Design review of the part built by this model. Coordinates are the model's own, in mm. A direction names the side the tool comes from. Coordinates: 2 decimals unless noted, no trailing zeros. Loops run counter-clockwise (first coordinate to the right, second up) from the corner with the lowest first, then second, coordinate; pieces in that order, holes last. Notation, with made-up numbers: (45, -33.5) -> (93, -33.5) arc R21 cw to (93, -4.5) -> close; hole circle Ø5 at (5, 40.5). An arc over 180 degrees is marked (long way). Use a Markdown table: item, result. Add a question column.
Q1. Take a section at B-B on y = -89.5. Write out the cut boundary in (x, z), plus the area to 3 significant figures.
Q2. Take a section at A-A on x = -114.5. Write out the cut boundary in (y, z), plus the area to 3 significant figures.
Q3. Clearance check with flat-ended pins moving along their axes: pin 1 Ø7 at (x, y) = (-122.68, -90.83) entering from -Z; pin 2 Ø7.5 at (y, z) = (-76.5, 57) entering from +X; pin 3 Ø1.5 at (x, z) = (-116.5, 21) entering from -Y; pin 4 Ø1.5 at (y, z) = (-89.5, 55.5) entering from +X. State where each tip first meets the part, or that it passes through.
Q4. For faces 4 (the face through (-111, -96.022, 39)), 5 (the face through (-127.874, -79, 39)), 6 (the face through (-123.036, -88.155, 39.44)), list the 3-axis set-ups (+Z, -Z, +X, -X, +Y, -Y) from which the entire face can be reached by the end or side of a thin tool; tool diameter is ignored.
Q5. For probe 1 along Y at (x, z) = (-122.75, 10.5); probe 2 along Y at (x, z) = (-111.75, 23); probe 3 along X at (y, z) = (-90, 36), list the stretches that pass through material, from the lowest coordinate up.
Q6. Take a section at D-D on x = -132.75. Write out the cut boundary in (y, z), plus the area to 3 significant figures.
Q7. Take a section at C-C on z = 11.5. Write out the cut boundary in (x, y), plus the area to 3 significant figures.
Q8. Draft analysis for pull direction Y (two halves, no side actions). For faces 1 (the face through (-132, -74.122, 39)), 2 (the face through (-115.974, -98, 39)), 3 (the face through (-121, -86, 0)), state which applies: pulls with the +Y half, pulls with the -Y half, needs draft (parallel to the pull), parting line crosses it, or undercut.
from build123d import *

# Parameters (mm, degrees)
F0_R        = 2.7
F1_DEPTH    = 80
F2_T1_DEPTH = 91.0076112648


# Not quite as in the source:
# - a fillet or chamfer that OpenCascade refuses, or shapes differently, is made with other operations: its cross-section is extruded or revolved along the edge and cut away or added


with BuildPart() as f1:
    # F0 (on Top) → F1 (new body)
    with BuildSketch(Plane.XY):
        with BuildLine():
            Line((-130.9739977717, -74.1217002273), (-135.9739977717, -74.1217002273))
            ThreePointArc((-135.9739977717, -74.1217002273), (-127.1872012073, -95.3349036629), (-105.9739977717, -104.1217002273))
            Line((-105.9739977717, -104.1217002273), (-105.9739977717, -99.1217002273))
            Line((-105.9739977717, -99.1217002273), (-115.4739977717, -99.1217002273))
            ThreePointArc((-115.4739977717, -99.1217002273), (-116.3275511623, -99.4752536179), (-115.9739977717, -98.6217002273))
            Line((-115.9739977717, -98.6217002273), (-115.9739977717, -96.5217002273))
            ThreePointArc((-115.9739977717, -96.5217002273), (-116.3275511623, -95.6681468367), (-115.4739977717, -96.0217002273))
            Line((-115.4739977717, -96.0217002273), (-105.9739977717, -96.0217002273))
            Line((-105.9739977717, -96.0217002273), (-105.9739977717, -95.0217002273))
            Line((-105.9739977717, -95.0217002273), (-126.8739977717, -74.1217002273))
            Line((-126.8739977717, -74.1217002273), (-127.8739977717, -74.1217002273))
            Line((-127.8739977717, -74.1217002273), (-127.8739977717, -83.6217002273))
            ThreePointArc((-127.8739977717, -83.6217002273), (-127.5204443811, -83.7681468367), (-127.3739977717, -84.1217002273))
            ThreePointArc((-127.3739977717, -84.1217002273), (-127.8739977717, -84.6217002273), (-128.3739977717, -84.1217002273))
            Line((-128.3739977717, -84.1217002273), (-130.4739977717, -84.1217002273))
            ThreePointArc((-130.4739977717, -84.1217002273), (-131.3275511623, -84.4752536179), (-130.9739977717, -83.6217002273))
            Line((-130.9739977717, -83.6217002273), (-130.9739977717, -74.1217002273))
        make_face()
        with Locations((-122.684560746, -90.8322632015)):
            Circle(F0_R, mode=Mode.SUBTRACT)
    extrude(amount=F1_DEPTH)

    # F2: chamfer of 2 on 2 edges, made by hand

    # F2_s2 → F2_t1 (cut)
    with BuildSketch(Plane.XY.offset(-5.5038056324)):
        with BuildLine():
            Line((-105.9739977717, -102.0501803148), (-108.1168549146, -104.0450717496))
            ThreePointArc((-108.1168549146, -104.0450717496), (-107.074368306, -104.1015131801), (-105.9739977717, -104.1217002273))
            Line((-105.9739977717, -104.1217002273), (-105.9739977717, -102.0501803148))
        make_face()
        with BuildLine():
            Line((-135.8973692941, -76.2645573701), (-133.9024778593, -74.1217002273))
            Line((-133.9024778593, -74.1217002273), (-135.9739977717, -74.1217002273))
            ThreePointArc((-135.9739977717, -74.1217002273), (-135.9538107246, -75.2220707615), (-135.8973692941, -76.2645573701))
        make_face()
    extrude(amount=F2_T1_DEPTH, mode=Mode.SUBTRACT)


solid = f1.part
Answer list:
| question | item | result |
|---|---|---|
| 1 | outline | (-131.73, 0) -> (-125.03, 0) -> (-125.03, 80) -> (-131.73, 80) -> close; (-120.34, 0) -> (-111.5, 0) -> (-111.5, 80) -> (-120.34, 80) -> close |
| 1 | area | 1,240 mm² |
| 2 | outline | (-102.88, 0) -> (-99.12, 0) -> (-99.12, 80) -> (-102.88, 80) -> close; (-96.02, 0) -> (-86.5, 0) -> (-86.5, 80) -> (-96.02, 80) -> close |
| 2 | area | 1,060 mm² |
| 3 | pin 1 | z = 0 |
| 3 | pin 2 | x = -120.75 |
| 3 | pin 3 | y = -102.48 |
| 3 | pin 4 | x = -110.75 |
| 4 | face 4 | +Z, -Z, +X |
| 4 | face 5 | +Z, -Z, +Y |
| 4 | face 6 | +Z, -Z |
| 5 | probe 1 | -98.99 to -93.53, -88.13 to -78.25 |
| 5 | probe 2 | -103.56 to -99.12, -96.02 to -89.25 |
| 5 | probe 3 | -131.43 to -125.25, -120.12 to -111 |
| 6 | outline | (-87.65, 0) -> (-74.12, 0) -> (-74.12, 80) -> (-87.65, 80) -> close |
| 6 | area | 1,080 mm² |
| 7 | outline | (-135.9, -76.26) arc R30 ccw to (-108.12, -104.05) -> (-105.97, -102.05) -> (-105.97, -99.12) -> (-115.47, -99.12) arc R0.5 cw (long way) to (-115.97, -98.62) -> (-115.97, -96.52) arc R0.5 cw (long way) to (-115.47, -96.02) -> (-105.97, -96.02) -> (-105.97, -95.02) -> (-126.87, -74.12) -> (-127.87, -74.12) -> (-127.87, -83.62) arc R0.5 cw (long way) to (-128.37, -84.12) -> (-130.47, -84.12) arc R0.5 cw (long way) to (-130.97, -83.62) -> (-130.97, -74.12) -> (-133.9, -74.12) -> close; hole circle Ø5.4 at (-122.68, -90.83) |
| 7 | area | 397 mm² |
| 8 | face 1 | pulls with the +Y half |
| 8 | face 2 | undercut |
| 8 | face 3 | needs draft |
